from build123d import *

# Parameters (mm, degrees)
EXTRUDE_1_DEPTH     = 2
EXTRUDE_2_DEPTH     = 3
SKETCH_4_W          = 1.7
SKETCH_4_H          = 2
CUT_EXTRUDE_1_DEPTH = 3.5


with BuildPart() as part:
    # Эскиз1 → Бобышка-Вытянуть1 (new body)
    with BuildSketch(Plane.XY):
        with BuildLine():
            Line((-0.15, -1.85), (0.15, -1.85))
            ThreePointArc((0.15, -1.85), (1.352081528, -1.352081528), (1.85, -0.15))
            Line((1.85, -0.15), (1.85, 0.15))
            ThreePointArc((1.85, 0.15), (1.352081528, 1.352081528), (0.15, 1.85))
            Line((0.15, 1.85), (-0.15, 1.85))
            ThreePointArc((-0.15, 1.85), (-1.352081528, 1.352081528), (-1.85, 0.15))
            Line((-1.85, 0.15), (-1.85, -0.15))
            ThreePointArc((-1.85, -0.15), (-1.352081528, -1.352081528), (-0.15, -1.85))
        make_face()
    extrude(amount=EXTRUDE_1_DEPTH)

    # Эскиз2 → Бобышка-Вытянуть2 (add)
    with BuildSketch(Plane.XY.offset(2)):
        with BuildLine():
            Line((-1.5, -3), (1.5, -3))
            ThreePointArc((1.5, -3), (2.560660172, -2.560660172), (3, -1.5))
            Line((3, -1.5), (3, 1.5))
            ThreePointArc((3, 1.5), (2.560660172, 2.560660172), (1.5, 3))
            Line((1.5, 3), (-1.5, 3))
            ThreePointArc((-1.5, 3), (-2.560660172, 2.560660172), (-3, 1.5))
            Line((-3, 1.5), (-3, -1.5))
            ThreePointArc((-3, -1.5), (-2.560660172, -2.560660172), (-1.5, -3))
        make_face()
    extrude(amount=EXTRUDE_2_DEPTH)

    # Эскиз4 → Вырез-Вытянуть1 (cut)
    with BuildSketch(Plane(origin=(0, 3, 0), x_dir=(1, 0, 0), z_dir=(0, 1, 0))):
        with Locations((0, -4)):
            Rectangle(SKETCH_4_W, SKETCH_4_H)
    extrude(amount=-CUT_EXTRUDE_1_DEPTH, mode=Mode.SUBTRACT)


solid = part.part
Read the model definition and answer for the solid it produces. Units are mm, in the model's axes. A direction names the side the tool comes from. Give positions to 0.01 mm unless a question says otherwise; leave off trailing zeros. Loops run counter-clockwise (first coordinate to the right, second up) from the corner with the lowest first, then second, coordinate; pieces in that order, holes last. Notation, with made-up numbers: (22.25, -17) -> (79.25, -17) arc R21 ccw to (79.25, -2) -> close; hole circle Ø4 at (55, -32). An arc over 180 degrees is marked (long way). Answer as CSV lines item,"result".
Item 1: Find section B-B on x = 0. Give the vertices of the cut face in (y, z), plus the area to 3 significant figures.
Returned:
outline,"(-3, 2) -> (-1.85, 2) -> (-1.85, 0) -> (1.85, 0) -> (1.85, 2) -> (3, 2) -> (3, 3) -> (-0.5, 3) -> (-0.5, 5) -> (-3, 5) -> close"
area,"18.4 mm²"
Item 2: Consider line 1 (X direction, y = 0.5, z = 4.25); line 2 (Z direction, x = -1.2, y = 1.6); line 3 (X direction, y = 2.4, z = 4.25). Determine where each line is inside the solid, lowest interval first. Write a range as [from, to].
Returned:
line 1,"x = [-3, -0.85], [0.85, 3]"
line 2,"z = [2, 5]"
line 3,"x = [-2.7, -0.85], [0.85, 2.7]"
Item 3: Find section C-C on z = 2.7. Give the vertices of the cut face in (x, y), plus the area to 3 significant figures.
Returned:
outline,"(-3, -1.5) arc R1.5 ccw to (-1.5, -3) -> (1.5, -3) arc R1.5 ccw to (3, -1.5) -> (3, 1.5) arc R1.5 ccw to (1.5, 3) -> (-1.5, 3) arc R1.5 ccw to (-3, 1.5) -> close"
area,"34.1 mm²"
Item 4: For faces 1 (the face through (-0.85, 1, 4)), 2 (the face through (1.3, -1.4, 1)), 3 (the face through (-1.3, 1.4, 1)), 4 (the face through (1.4, 1.3, 1)), determine the directions among +Z, -Z, +X, -X, +Y, -Y from which every point of the face is accessible in a straight line to the end or side of a thin tool.
Returned:
face 1,"+Z, +Y"
face 2,"-Z, +X, -Y"
face 3,"-Z, -X, +Y"
face 4,"-Z, +X, +Y"
Item 5: Determine the mould class of faces 5 (the face through (0.85, 1, 4)), 6 (the face through (0, 3, 2.8)), 7 (the face through (2.57, 2.55, 3.48)), 8 (the face through (0, -0.5, 4)) for opening direction X: +X half, -X half, draft (parallel to the pull), parting line (faces both ways), or undercut.
Returned:
face 5,"undercut"
face 6,"draft"
face 7,"+X half"
face 8,"undercut"
Item 6: Each of these flat-tipped pins is pushed along its axis until it touches: pin 1 (1 mm diameter, centred on y = 2.5, z = 3.5, fed in from -X); pin 2 (0.8 mm diameter, centred on x = 0, y = 0.5, fed in from +Z). Where does it stop, or does it pass through?
Returned:
pin 1,"stops at x = -2.91"
pin 2,"stops at z = 3"
Item 7: Find section D-D on y = 0.95. Give the vertices of the cut face in (x, z), plus the area to 3 significant figures.
Returned:
outline,"(-3, 2) -> (-1.65, 2) -> (-1.65, 0) -> (1.65, 0) -> (1.65, 2) -> (3, 2) -> (3, 5) -> (0.85, 5) -> (0.85, 3) -> (-0.85, 3) -> (-0.85, 5) -> (-3, 5) -> close"
area,"21.2 mm²"
Item 8: Find section A-A on y = 0. Give the vertices of the cut face in (x, z).
Returned:
outline,"(-3, 2) -> (-1.85, 2) -> (-1.85, 0) -> (1.85, 0) -> (1.85, 2) -> (3, 2) -> (3, 5) -> (0.85, 5) -> (0.85, 3) -> (-0.85, 3) -> (-0.85, 5) -> (-3, 5) -> close"
